Source: CAD feature listing. Evaluate the final solid. Frame: model axes, mm. Face numbers are marked on the shaded views. A direction names the side the tool comes from. Give positions to 0.01 mm unless a question says otherwise; leave off trailing zeros. Order: outer loops, then holes, each group sorted by start corner. A loop starts at its lowest first (then second) coordinate and runs counter-clockwise, first axis right, second up.
from build123d import *

# Parameters (mm, degrees)
F1_DEPTH = 1.6
F3_DEPTH = 20
F5_DEPTH = 34.001
F6_W     = 34
F6_H     = 34
F6_W_2   = 30.5
F6_H_2   = 30.5
F7_DEPTH = 10
F6_R     = 8
F8_DEPTH = 16.7997198341


# Not quite as in the source:
# - a feature names something its author has since deleted; it is built from what else it names


with BuildPart() as f1:
    # F0 (on Top) → F1 (new body)
    with BuildSketch(Plane.XY):
        Polygon((-15.7, 19), (-17, 19), (-17, -19), (-15.7, -19), (-15.7, -20.5), (-6.7, -20.5), (-6.7, -19), (6.7, -19), (6.7, -20.5), (15.7, -20.5), (15.7, -19), (17, -19), (17, 19), (15.7, 19), (15.7, 20.5), (6.7, 20.5), (6.7, 19), (-6.7, 19), (-6.7, 20.5), (-15.7, 20.5), align=None)
    extrude(amount=F1_DEPTH)

    # F2 (on face) → F3 (join)
    with BuildSketch(Plane.XY.offset(1.6)):
        Polygon((-15.7, 19), (-17, 19), (-17, -19), (-15.7, -19), (-6.7, -19), (6.7, -19), (15.7, -19), (17, -19), (17, 19), (15.7, 19), (6.7, 19), (-6.7, 19), align=None)
    extrude(amount=F3_DEPTH)

    # F4 (on face) → F5 (cut, through all)
    with BuildSketch(Plane(origin=(-17, 0, 0), x_dir=(0, -1, 0), z_dir=(-1, 0, 0))):
        Polygon((-19, 17.3308689021), (19, 3.5), (19, 21.6), (-19, 21.6), align=None)
    extrude(amount=-F5_DEPTH, mode=Mode.SUBTRACT)

    # F6 (on face) → F7 (join)
    with BuildSketch(Plane(origin=(0, -3.3474561073, 9.1970600675), x_dir=(1, 0, 0), z_dir=(0, -0.3420201433, 0.9396926208))):
        with Locations((0, 4.0929107067)):
            Rectangle(F6_W, F6_H)
        with Locations((0, 4.0929107067)):
            Rectangle(F6_W_2, F6_H_2, mode=Mode.SUBTRACT)
    extrude(amount=F7_DEPTH)

    # F6 (on face) → F8 (cut, through all)
    with BuildSketch(Plane(origin=(0, -3.3474561073, 9.1970600675), x_dir=(1, 0, 0), z_dir=(0, -0.3420201433, 0.9396926208))):
        with Locations((0, 4.0929107067)):
            Circle(F6_R)
    extrude(amount=-F8_DEPTH, mode=Mode.SUBTRACT)


solid = f1.part
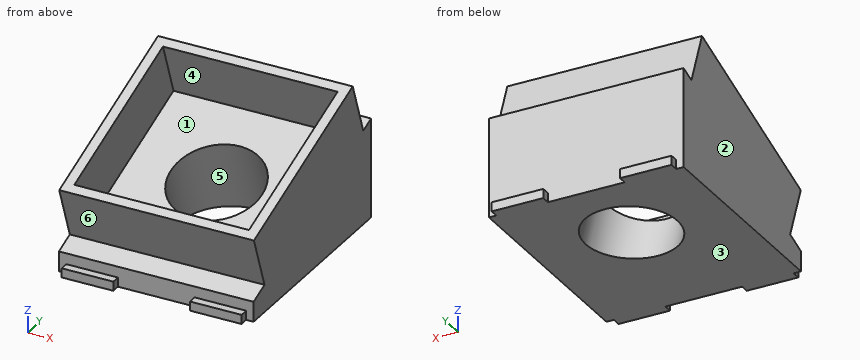
1) Section query B-B on x = 0. Output: boundary loops of the cut face in (y, z).
Checks:
outline: (-19, 0) - (-4.16, 0) - (-7.02, 7.86) - (-13.83, 5.38) - (-17.25, 14.78) - (-18.9, 14.18) - (-15.48, 4.78) - (-19, 3.5) - close; (8.02, 13.33) - (12.87, 0) - (19, 0) - (19, 17.33) - (16.47, 16.41) - (13.05, 25.81) - (11.41, 25.21) - (14.83, 15.81) - close
2) Reachability of the marked faces 4, 5 and 6 from +Z, -Z, +X, -X, +Y, -Y: full face, straight path, thin tool, end or side. Return the list, or none.
Checks:
face 4: -Y
face 5: none
face 6: +X, -X, -Y
3) First-contact query: pin 1 Ø0.8 at (y, z) = (19.5, 1) entering from +X; pin 2 Ø0.8 at (y, z) = (19.5, 0.5) entering from -X; pin 3 Ø2 at (x, y) = (7.5, 12) entering from +Z. Flat tips, straight axial feed; report the tip coordinate or a pass-through.
Checks:
pin 1: stops at x = 15.7
pin 2: stops at x = -15.7
pin 3: stops at z = 25.79
4) Section query D-D on z = 19.25. Output: boundary loops of the cut face in (x, y).
Checks:
outline: (-17, -4.97) - (-15.25, -4.97) - (-15.25, 13.58) - (15.25, 13.58) - (15.25, -4.97) - (17, -4.97) - (17, 15.44) - (-17, 15.44) - close
5) Pull-direction query (Z, two-part tool) for the marked faces 1, 2 and 3; classes: +Z half, -Z half, draft (parallel to the pull), parting line (faces both ways), or undercut.
Checks:
face 1: undercut
face 2: draft
face 3: -Z half
6) Section query C-C on y = -8.5. Output: boundary loops of the cut face in (x, z).
Checks:
outline: (-17, 0) - (17, 0) - (17, 17.96) - (15.25, 17.96) - (15.25, 7.32) - (-15.25, 7.32) - (-15.25, 17.96) - (-17, 17.96) - close
7) Ray query, L1, parallel to X at y = -3.5, z = 8.75; L2, parallel to X at y = -11, z = 8; L3, parallel to Z at x = -7, y = -3.5. Return the intervals inside material, ascending.
Checks:
L1: x = -17 to -6.69, 6.69 to 17
L2: x = -17 to -15.25, 15.25 to 17
L3: z = 0 to 9.14
8) Section query A-A on x = -13.5. Output: boundary loops of the cut face in (y, z).
Checks:
outline: (-20.5, 0) - (20.5, 0) - (20.5, 1.6) - (19, 1.6) - (19, 17.33) - (16.47, 16.41) - (13.05, 25.81) - (11.41, 25.21) - (14.83, 15.81) - (-13.83, 5.38) - (-17.25, 14.78) - (-18.9, 14.18) - (-15.48, 4.78) - (-19, 3.5) - (-19, 1.6) - (-20.5, 1.6) - close
